CAD build for the part. Positions are in the model's coordinates, mm. A direction names the side the tool comes from. Round coordinates to 2 decimals unless told otherwise and drop trailing zeros. Write each loop counter-clockwise with the first axis right and the second up, starting at its lowest first coordinate (ties: lowest second). Pieces come first, ordered by that corner, then holes. Notation, with made-up numbers: (16, 70.25) - (48, 70.25) arc R31 cw to (48, 108.25) - close; hole circle Ø10 at (-30, 53.5). An arc over 180 degrees is marked (long way). Answer in a Markdown table with one row per item.
```python
from build123d import *

# Parameters (mm, degrees)
SKETCH_1_W      = 30
SKETCH_1_H      = 100
SKETCH_1_W_2    = 10
SKETCH_1_H_2    = 10
EXTRUDE_1_DEPTH = 10
SKETCH_2_W      = 10
SKETCH_2_H      = 10.013991437
EXTRUDE_2_DEPTH = 50
SKETCH_3_W      = 120
SKETCH_3_H      = 10
SKETCH_3_R      = 2.5
EXTRUDE_3_DEPTH = 10


with BuildPart() as part:
    # 스케치1 → 보스-돌출1 (new body)
    with BuildSketch(Plane.XY):
        Rectangle(SKETCH_1_W, SKETCH_1_H)
        with Locations((0, 10)):
            Rectangle(SKETCH_1_W_2, SKETCH_1_H_2, mode=Mode.SUBTRACT)
        with Locations((0, 30)):
            Rectangle(SKETCH_1_W_2, SKETCH_1_H_2, mode=Mode.SUBTRACT)
        with Locations((0, -10)):
            Rectangle(SKETCH_1_W_2, SKETCH_1_H_2, mode=Mode.SUBTRACT)
        with Locations((0, -30)):
            Rectangle(SKETCH_1_W_2, SKETCH_1_H_2, mode=Mode.SUBTRACT)
    extrude(amount=EXTRUDE_1_DEPTH)

    # 스케치2 → 보스-돌출2 (add)
    with BuildSketch(Plane(origin=(15, 0, 0), x_dir=(0, 0, -1), z_dir=(1, 0, 0))):
        with Locations((-5, -44.993004282)):
            Rectangle(SKETCH_2_W, SKETCH_2_H)
    extrude(amount=EXTRUDE_2_DEPTH)

    # 스케치3 → 보스-돌출3 (add)
    with BuildSketch(Plane(origin=(65, 0, 0), x_dir=(0, 0, -1), z_dir=(1, 0, 0))):
        with Locations((-60, -44.986008563)):
            Rectangle(SKETCH_3_W, SKETCH_3_H)
        with Locations((-115, -44.986008563)):
            Circle(SKETCH_3_R, mode=Mode.SUBTRACT)
    extrude(amount=-EXTRUDE_3_DEPTH)


solid = part.part
```
Q1. Pull direction X, two halves, no side cores. Call faces 4 (the flat face through (5, -10, 5)), 5 (the flat face through (13, -8, 0)), 6 (the flat face through (15, 4, 5)), 7 (the flat face through (55, -45, 66)): released by +X, released by -X, zero draft, split by the parting line, or undercut.
Computed:
| item | result |
|---|---|
| face 4 | undercut |
| face 5 | zero draft |
| face 6 | released by +X |
| face 7 | released by -X |
Q2. Saw through at B-B on x = 7. List the corners of the cut face in (y, z).
Computed:
| item | result |
|---|---|
| outline | (-50, 0) - (50, 0) - (50, 10) - (-50, 10) - close |
Q3. Drill centre lines: line 1 (Y direction, x = 58, z = 115); line 2 (Y direction, x = 59, z = 101); line 3 (Z direction, x = -1, y = -18). Where is each one in solid material? Low to high.
Computed:
| item | result |
|---|---|
| line 1 | y = -49.99 to -47.49, -42.49 to -39.99 |
| line 2 | y = -49.99 to -39.99 |
| line 3 | z = 0 to 10 |
Q4. Flat gauge pins, fed straight in: pin 1 (4 mm diameter, centred on y = -44.99, z = 115, fed in from -X); pin 2 (5 mm diameter, centred on y = -9, z = 5.5, fed in from +X); pin 3 (10 mm diameter, centred on x = -4, y = 38, fed in from +Z). Where does each tip first touch, or does it go through?
Computed:
| item | result |
|---|---|
| pin 1 | passes through |
| pin 2 | stops at x = 15 |
| pin 3 | stops at z = 10 |
Q5. Saw through at A-A on z = 115. List the corners of the cut face in (x, y), then the cut area to 3 significant figures.
Computed:
| item | result |
|---|---|
| outline | (55, -49.99) - (65, -49.99) - (65, -47.49) - (55, -47.49) - close; (55, -42.49) - (65, -42.49) - (65, -39.99) - (55, -39.99) - close |
| area | 50.0 mm2 |
Q6. Saw through at C-C on y = -1.5. List the corners of the cut face in (x, z), then the cut area to 3 significant figures.
Computed:
| item | result |
|---|---|
| outline | (-15, 0) - (15, 0) - (15, 10) - (-15, 10) - close |
| area | 300 mm2 |
Q7. 3-axis set-ups, long thin cutter, end or side, ignore diameter. For faces 1 (the flat face through (5, 10, 5)), 2 (the flat face through (60, -45, 120)), 3 (the flat face through (7, -8, 10)): which of +Z, -Z, +X, -X, +Y, -Y reach the whole face in a straight line?
Computed:
| item | result |
|---|---|
| face 1 | +Z, -Z |
| face 2 | +Z, +X, -X, +Y, -Y |
| face 3 | +Z, -X, +Y, -Y |
